```python
from build123d import *

# Parameters (mm, degrees)
CROQUIS1_W                                 = 56.1
CROQUIS1_H                                 = 56.1
SALIENTE_EXTRUIR1_DEPTH                    = 76.05
CORTAR_EXTRUIR1_DEPTH                      = 82.199307263
SIMETR_A3_AT_THE_SECOND_PLANE_COPY_1_DEPTH = 82.199307263
CHAFL_N1_SIZE                              = 2.5
CROQUIS3_R                                 = 2.25
CORTAR_EXTRUIR2_DEPTH                      = 82.199307263
SIMETR_A4_AT_THE_SECOND_PLANE_COPY_1_SKE_R = 2.25
SIMETR_A4_AT_THE_SECOND_PLANE_COPY_1_DEPTH = 82.199307263
CROQUIS4_R                                 = 19.25
CORTAR_EXTRUIR3_DEPTH                      = 2.5


with BuildPart() as part:
    # Croquis1 → Saliente-Extruir1 (new body)
    with BuildSketch(Plane(origin=(0, 0, 0), x_dir=(1, 0, 0), z_dir=(0, 1, 0))):
        Rectangle(CROQUIS1_W, CROQUIS1_H)
    extrude(amount=SALIENTE_EXTRUIR1_DEPTH)

    # Croquis2 → Cortar-Extruir1 (cut, through all)
    with BuildSketch(Plane(origin=(0, 70.85, 0), x_dir=(1, 0, 0), z_dir=(0, 1, 0))):
        with BuildLine():
            Line((-28.05, 19.7), (-23.875, 19.7))
            ThreePointArc((-23.875, 19.7), (-20.922829189, 20.922829189), (-19.7, 23.875))
            Line((-19.7, 23.875), (-19.7, 28.05))
            Line((-19.7, 28.05), (-28.05, 28.05))
            Line((-28.05, 28.05), (-28.05, 19.7))
        make_face()
    cortar_extruir1 = extrude(amount=-CORTAR_EXTRUIR1_DEPTH, mode=Mode.SUBTRACT)

    # Simetría3: Cortar-Extruir1 across plane
    add(cortar_extruir1.mirror(Plane(origin=(0, 0, 0), x_dir=(0, 0, 1), z_dir=(1, 0, 0))), mode=Mode.SUBTRACT)

    # Simetría3 at the second plane: Cortar-Extruir1 across plane
    add(cortar_extruir1.mirror(Plane.XY), mode=Mode.SUBTRACT)

    # Simetría3 at the second plane copy 1 ske → Simetría3 at the second plane copy 1 (cut, through all)
    with BuildSketch(Plane(origin=(0, 70.85, 0), x_dir=(-1, 0, 0), z_dir=(0, 1, 0))):
        with BuildLine():
            Line((-28.05, 19.7), (-23.875, 19.7))
            ThreePointArc((-23.875, 19.7), (-20.922829189, 20.922829189), (-19.7, 23.875))
            Line((-19.7, 23.875), (-19.7, 28.05))
            Line((-19.7, 28.05), (-28.05, 28.05))
            Line((-28.05, 28.05), (-28.05, 19.7))
        make_face()
    extrude(amount=-SIMETR_A3_AT_THE_SECOND_PLANE_COPY_1_DEPTH, mode=Mode.SUBTRACT)

    # Chaflán1
    chafl_n1_edges = [part.edges().sort_by_distance(p)[0] for p in [
        (-28.05, 35.425, -19.7),
        (-19.7, 35.425, -28.05),
        (-28.05, 35.425, 19.7),
        (-19.7, 35.425, 28.05),
        (28.05, 35.425, -19.7),
        (19.7, 35.425, -28.05),
        (28.05, 35.425, 19.7),
        (19.7, 35.425, 28.05),
    ]]
    chamfer(chafl_n1_edges, length=CHAFL_N1_SIZE)

    # Croquis3 → Cortar-Extruir2 (cut, through all)
    with BuildSketch(Plane.XZ.offset(-70.85)):
        with Locations(Location((23.875, -23.875, 0), (0, 0, 270))):
            Circle(CROQUIS3_R)
    cortar_extruir2 = extrude(amount=-CORTAR_EXTRUIR2_DEPTH, mode=Mode.SUBTRACT)

    # Simetría4: Cortar-Extruir2 across plane
    add(cortar_extruir2.mirror(Plane(origin=(0, 0, 0), x_dir=(0, 0, 1), z_dir=(1, 0, 0))), mode=Mode.SUBTRACT)

    # Simetría4 at the second plane: Cortar-Extruir2 across plane
    add(cortar_extruir2.mirror(Plane.XY), mode=Mode.SUBTRACT)

    # Simetría4 at the second plane copy 1 ske → Simetría4 at the second plane copy 1 (cut, through all)
    with BuildSketch(Plane(origin=(0, 70.85, 0), x_dir=(-1, 0, 0), z_dir=(0, -1, 0))):
        with Locations(Location((23.875, -23.875, 0), (0, 0, 270))):
            Circle(SIMETR_A4_AT_THE_SECOND_PLANE_COPY_1_SKE_R)
    extrude(amount=-SIMETR_A4_AT_THE_SECOND_PLANE_COPY_1_DEPTH, mode=Mode.SUBTRACT)

    # Croquis4 → Cortar-Extruir3 (cut)
    with BuildSketch(Plane(origin=(0, 76.05, 0), x_dir=(1, 0, 0), z_dir=(0, 1, 0))):
        with Locations(Location((0, 0, 0), (0, 0, 270))):
            Circle(CROQUIS4_R)
    extrude(amount=-CORTAR_EXTRUIR3_DEPTH, mode=Mode.SUBTRACT)


solid = part.part
```
CAD build for the part. Positions are in the model's coordinates, mm. A direction names the side the tool comes from. Coordinates: 2 decimals unless noted, no trailing zeros. Write each loop counter-clockwise with the first axis right and the second up, starting at its lowest first coordinate (ties: lowest second). Pieces come first, ordered by that corner, then holes. Notation, with made-up numbers: (-24.5, 77.5) -> (23.5, 77.5) arc R18 ccw to (23.5, 99.5) -> close; hole circle Ø11 at (57, 83). An arc over 180 degrees is marked (long way). Use CSV: the item, a comma, the result in double quotes. Start each with the question number.
Item 1: Band-saw the part on C-C, the plane z = 0. Write the cut outline in (x, y), plus the area to 3 significant figures.
Item 2: Drop flat-ended pins along their axis: P1, Ø1, axis at y = 47, z = -19.5, coming from the +X side; P2, Ø1.8, axis at x = 24.5, y = 30.5, coming from the -Z side; P3, Ø5.5, axis at x = -23, z = 24.5, coming from the -Y side; P4, Ø3.5, axis at x = -23.875, z = -23.875, coming from the +Y side. Give the stop position or say it passes through.
Item 3: Band-saw the part on B-B, the plane x = 0. Write the cut outline in (y, z).
Item 4: Tool access for faces 1 (the flat face through (25, 36, 19.7)), 2 (the flat face through (-25, 36, 19.7)), 3 (the flat face through (25, 36, -19.7)), 4 (the flat face through (-18.47, 35.92, -26.78)): list every direction of +Z, -Z, +X, -X, +Y, -Y with a clear straight run to the whole face (end or side of a thin tool).
Item 5: Two-plate mould, pull along X, no slides. Class faces 5 (the cylindrical face through (21.879, 73.414, 24.913)), 6 (the flat face through (-23.9, 70.85, 26.3)), 7 (the flat face through (-19.7, 36, 25)), 8 (the flat face through (26.78, 35.92, 18.47)): +X half, -X half, draft (parallel to the pull), parting line (faces both ways), or undercut.
Item 6: Wall check: probe 1 along Y at (x, z) = (16, -8); probe 2 along X at (y, z) = (30.5, -26); probe 3 along Z at (x, y) = (24, 10). Give the ranges that are in metal, low to high.
Item 7: Band-saw the part on A-A, the plane y = 54.5. Write the cut outline in (x, z) (3 decimals).
Response values:
1,outline,"(-28.05, 0) -> (28.05, 0) -> (28.05, 76.05) -> (19.25, 76.05) -> (19.25, 73.55) -> (-19.25, 73.55) -> (-19.25, 76.05) -> (-28.05, 76.05) -> close"
1,area,"4,170 mm2"
2,P1,"stops at x = 26.25"
2,P2,"stops at z = -19.71"
2,P3,"stops at y = 70.85"
2,P4,"passes through"
3,outline,"(0, -28.05) -> (76.05, -28.05) -> (76.05, -19.25) -> (73.55, -19.25) -> (73.55, 19.25) -> (76.05, 19.25) -> (76.05, 28.05) -> (0, 28.05) -> close"
4,face 1,"+Z, +X, -Y"
4,face 2,"+Z, -X, -Y"
4,face 3,"-Z, +X, -Y"
4,face 4,"-Z, -X, -Y"
5,face 5,"undercut"
5,face 6,"draft"
5,face 7,"-X half"
5,face 8,"+X half"
6,probe 1,"y = 0 to 73.55"
6,probe 2,"x = -19.25 to 19.25"
6,probe 3,"z = -19.7 to 19.7"
7,outline,"(-28.05, -17.2) -> (-25.55, -19.7) -> (-23.875, -19.7) arc R4.175 cw to (-19.7, -23.875) -> (-19.7, -25.55) -> (-17.2, -28.05) -> (17.2, -28.05) -> (19.7, -25.55) -> (19.7, -23.875) arc R4.175 cw to (23.875, -19.7) -> (25.55, -19.7) -> (28.05, -17.2) -> (28.05, 17.2) -> (25.55, 19.7) -> (23.875, 19.7) arc R4.175 cw to (19.7, 23.875) -> (19.7, 25.55) -> (17.2, 28.05) -> (-17.2, 28.05) -> (-19.7, 25.55) -> (-19.7, 23.875) arc R4.175 cw to (-23.875, 19.7) -> (-25.55, 19.7) -> (-28.05, 17.2) -> close"
